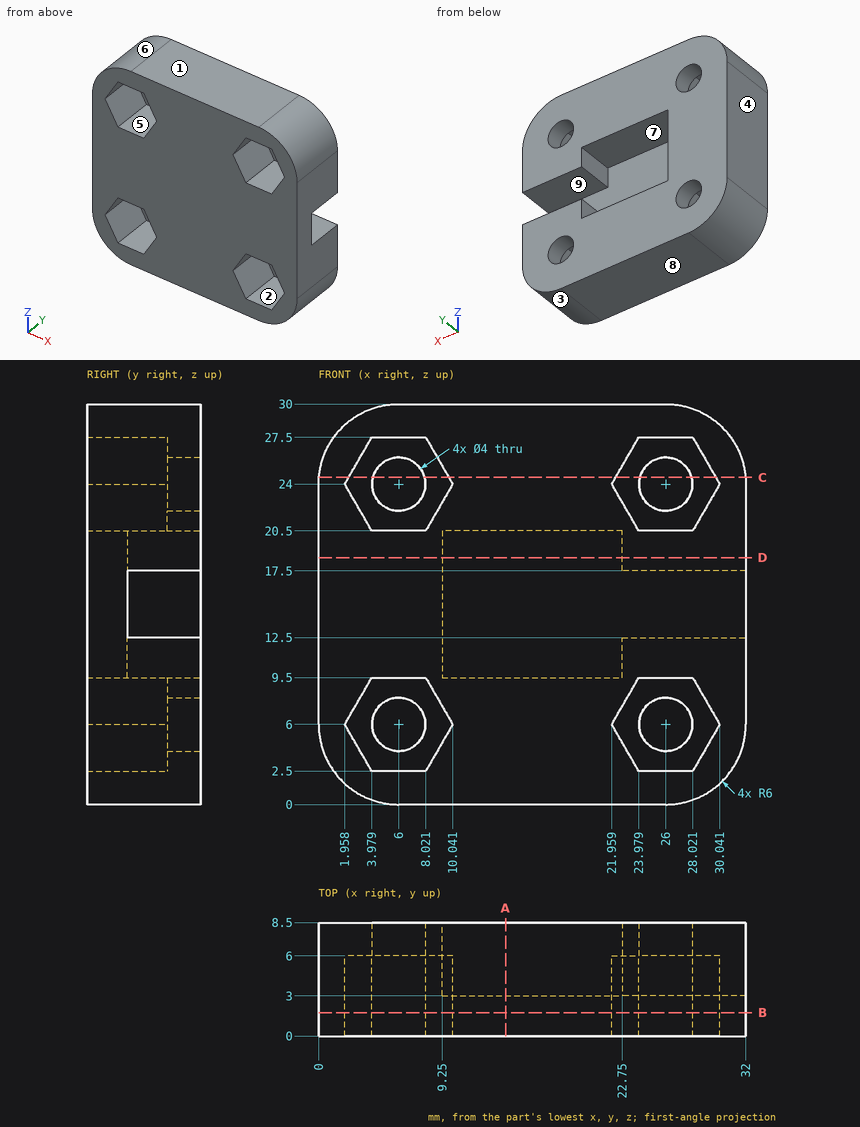
Geometry: see drawing. Coordinates: mm, zero at the bounding-box minimum. A direction names the side the tool comes from. Give positions to 0.01 mm unless a question says otherwise; leave off trailing zeros. Order: outer loops, then holes, each group sorted by start corner. A loop starts at its lowest first (then second) coordinate and runs counter-clockwise, first axis right, second up.
1. Pin query (flat end, axial travel): pin 1 Ø3.5 at (x, z) = (27.5, 24.5) entering from -Y. Return the tip coordinate at first contact, or that it passes through.
Computed:
pin 1: stops at y = 6
2. Cut plane C-C (z = 24.5). Return loops of the section in (x, y).
Computed:
outline: (0.02, 0) - (2.25, 0) - (2.25, 6) - (4.06, 6) - (4.06, 8.5) - (0.02, 8.5) - close; (7.94, 6) - (9.75, 6) - (9.75, 0) - (22.25, 0) - (22.25, 6) - (24.06, 6) - (24.06, 8.5) - (7.94, 8.5) - close; (27.94, 6) - (29.75, 6) - (29.75, 0) - (31.98, 0) - (31.98, 8.5) - (27.94, 8.5) - close
3. Draft query along X for the marked faces 1, 2, 3 and 4. Return one class per face: released by +X, released by -X, zero draft, split by the parting line, or undercut.
Computed:
face 1: zero draft
face 2: undercut
face 3: released by +X
face 4: released by -X
4. Cut plane B-B (y = 1.75). State how many separate pieces and enclosed holes the cut face has.
Computed:
separate pieces: 1
enclosed holes: 4
5. Set-up query: the marked faces 5, 6, 7, 8 and 9. Return all of +Z, -Z, +X, -X, +Y, -Y with unobstructed straight access to the full face (end or side cutting, diameter ignored); none if empty.
Computed:
face 5: -Y
face 6: +Z, -X, +Y, -Y
face 7: +Y
face 8: -Z, +X, -X, +Y, -Y
face 9: +X, +Y
6. Line query: probe 1 along X at (y, z) = (6.65, 6); probe 2 along Z at (x, y) = (26, 6.9); probe 3 along Z at (x, y) = (6, 8). Output: solid intervals per line, ascending.
Computed:
probe 1: x = 0 to 4, 8 to 24, 28 to 32
probe 2: z = 0 to 4, 8 to 12.5, 17.5 to 22, 26 to 30
probe 3: z = 0 to 4, 8 to 22, 26 to 30
7. Cut plane D-D (z = 18.5). Return loops of the section in (x, y), and give its area (3 significant figures).
Computed:
outline: (0, 0) - (32, 0) - (32, 8.5) - (22.75, 8.5) - (22.75, 3) - (9.25, 3) - (9.25, 8.5) - (0, 8.5) - close
area: 198 mm2
8. Cut plane A-A (x = 14). Return loops of the section in (y, z).
Computed:
outline: (0, 0) - (8.5, 0) - (8.5, 9.5) - (3, 9.5) - (3, 20.5) - (8.5, 20.5) - (8.5, 30) - (0, 30) - close
